For this review, take the finished solid that the model builds, in its own axes (mm). A direction names the side the tool comes from. Round coordinates to 2 decimals unless told otherwise and drop trailing zeros. Loops run counter-clockwise (first coordinate to the right, second up) from the corner with the lowest first, then second, coordinate; pieces in that order, holes last. Notation, with made-up numbers: (42, 23) -> (60, 23) arc R3 ccw to (60, 27) -> close; hole circle Ø3 at (27, 23.5). An arc over 180 degrees is marked (long way). Use one line per item in the form item = value. Start each with the question number.
from build123d import *

# Parameters (mm, degrees)
SKETCH1_W           = 40
SKETCH1_H           = 40
BOSS_EXTRUDE1_DEPTH = 40
SKETCH4_W           = 40
SKETCH4_H           = 40
CUT_EXTRUDE1_DEPTH  = 5
SKETCH5_W           = 40
SKETCH5_H           = 40
CUT_EXTRUDE2_DEPTH  = 5
SKETCH6_W           = 40
SKETCH6_H           = 40
CUT_EXTRUDE3_DEPTH  = 5
FILLET1_R           = 5
BOSS_EXTRUDE2_START = 5
BOSS_EXTRUDE2_DEPTH = 5
FILLET2_R           = 2.5
BOSS_EXTRUDE3_DEPTH = 0.1


with BuildPart() as part:
    # Sketch1 → Boss-Extrude1 (new body)
    with BuildSketch(Plane(origin=(0, 0, 0), x_dir=(0, 1, 0), z_dir=(0, 0, 1))):
        with Locations((20, -20)):
            Rectangle(SKETCH1_W, SKETCH1_H)
    extrude(amount=BOSS_EXTRUDE1_DEPTH)

    # Sketch2 → Cut-Revolve1 (revolve, cut)
    with BuildSketch(Plane.XZ):
        with BuildLine():
            Line((0, 42), (0, -42))
            ThreePointArc((0, -42), (42, 0), (0, 42))
        make_face()
    revolve(axis=Axis((0, 0, 42), (0, 0, -1)), mode=Mode.SUBTRACT)

    # Sketch4 → Cut-Extrude1 (cut)
    with BuildSketch(Plane.XZ):
        with Locations((20, 20)):
            Rectangle(SKETCH4_W, SKETCH4_H)
    extrude(amount=-CUT_EXTRUDE1_DEPTH, mode=Mode.SUBTRACT)

    # Sketch5 → Cut-Extrude2 (cut)
    with BuildSketch(Plane(origin=(0, 0, 0), x_dir=(0, -1, 0), z_dir=(-1, 0, 0))):
        with Locations((-20, 20)):
            Rectangle(SKETCH5_W, SKETCH5_H)
    extrude(amount=-CUT_EXTRUDE2_DEPTH, mode=Mode.SUBTRACT)

    # Sketch6 → Cut-Extrude3 (cut)
    with BuildSketch(Plane(origin=(0, 0, 0), x_dir=(1, 0, 0), z_dir=(0, 0, -1))):
        with Locations((20, -20)):
            Rectangle(SKETCH6_W, SKETCH6_H)
    extrude(amount=-CUT_EXTRUDE3_DEPTH, mode=Mode.SUBTRACT)

    # Fillet1
    fillet1_edges = [part.edges().sort_by_distance(p)[0] for p in [
        (22.5, 40, 40),
        (40, 22.5, 40),
        (40, 40, 22.5),
    ]]
    fillet(fillet1_edges, radius=FILLET1_R)

    # Sketch7 → Boss-Extrude2 (add)
    with BuildSketch(Plane.XZ.offset(-5).offset(BOSS_EXTRUDE2_START)):
        with BuildLine():
            Line((31.464466094, 40), (31.464466094, 35))
            Line((31.464466094, 35), (35, 31.464466094))
            Line((35, 31.464466094), (40, 31.464466094))
            Line((40, 31.464466094), (40, 35))
            ThreePointArc((40, 35), (38.535533906, 38.535533906), (35, 40))
            Line((35, 40), (31.464466094, 40))
        make_face()
    boss_extrude2 = extrude(amount=-BOSS_EXTRUDE2_DEPTH)

    # Mirror1: Boss-Extrude2 across plane
    add(boss_extrude2.mirror(Plane(origin=(0, 0, 0), x_dir=(0, 0.7071067811865476, 0.7071067811865476), z_dir=(0, 0.7071067811865477, -0.7071067811865475))))

    # Mirror1 at the second plane: Boss-Extrude2 across plane
    add(boss_extrude2.mirror(Plane(origin=(0, 0, 0), x_dir=(0, 0, 1), z_dir=(-0.7071067811865476, 0.7071067811865475, 0))))

    # Fillet2
    fillet2_edges = [part.edges().sort_by_distance(p)[0] for p in [
        (38.535533906, 0, 38.535533906),
        (33.232233047, 0, 40),
        (40, 0, 33.232233047),
        (0, 38.535533906, 38.535533906),
        (0, 40, 33.232233047),
        (0, 33.232233047, 40),
        (38.535533906, 38.535533906, 0),
        (40, 33.232233047, 0),
        (33.232233047, 40, 0),
    ]]
    fillet(fillet2_edges, radius=FILLET2_R)

    # Sketch9 → Boss-Extrude3 (add)
    with BuildSketch(Plane.YZ.offset(40)):
        with BuildLine():
            Line((32.5, 35), (5, 35))
            ThreePointArc((5, 35), (3.232233047, 34.267766953), (2.5, 32.5))
            Line((2.5, 32.5), (2.5, 10))
            ThreePointArc((2.5, 10), (4.696699141, 4.696699141), (10, 2.5))
            Line((10, 2.5), (32.5, 2.5))
            ThreePointArc((32.5, 2.5), (34.267766953, 3.232233047), (35, 5))
            Line((35, 5), (35, 32.5))
            ThreePointArc((35, 32.5), (34.267766953, 34.267766953), (32.5, 35))
        make_face()
    boss_extrude3 = extrude(amount=BOSS_EXTRUDE3_DEPTH)

    # Mirror2: Boss-Extrude3 across plane
    add(boss_extrude3.mirror(Plane(origin=(0, 0, 0), x_dir=(0.7071067811865475, 0, 0.7071067811865476), z_dir=(0.7071067811865478, 0, -0.7071067811865474))))

    # Mirror2 at the second plane: Boss-Extrude3 across plane
    add(boss_extrude3.mirror(Plane(origin=(0, 0, 0), x_dir=(0, 0, 1), z_dir=(-0.7071067811865476, 0.7071067811865475, 0))))


solid = part.part
Item 1: Wall thickness on line 1 (X direction, y = 29.5, z = 34); line 2 (Z direction, x = 34, y = 35); line 3 (X direction, y = 20.5, z = 7): over which ranges is each line inside the solid? List them lowest first.
Item 2: Machinability: for faces 1 (the flat face through (40, 34.4, 3)), 2 (the flat face through (31, 31, 5)), 3 (the flat face through (3.1, 34.5, 40)), 4 (the flat face through (40, 34.5, 34.5)), which of the approach directions +Z, -Z, +X, -X, +Y, -Y give a long, thin tool a straight path to every point of the face, cutting with its end or side? Answer none if there is none.
Item 3: Draft analysis for pull direction Y (two halves, no side actions). For faces 5 (the flat face through (31.464, 38, 2)), 6 (the flat face through (34, 0, 35)), 7 (the cylindrical face through (33.207, 39.287, 0.752)), state which applies: +Y half, -Y half, draft (parallel to the pull), parting line (faces both ways), or undercut.
Item 4: Take a section at B-B on y = 24. Give the boundary of the cut face in (x, z), plus the area to 3 significant figures.
Item 5: Take a section at A-A on z = 7. Give the boundary of the cut face in (x, y).
Item 6: Take a section at D-D on x = 9. Give the boundary of the cut face in (y, z), plus the area to 3 significant figures.
Item 7: Take a section at C-C on x = 15. Give the boundary of the cut face in (y, z), plus the area to 3 significant figures.
Item 8: For P1, Ø10, axis at x = 22, y = 12, coming from the -Z side; P2, Ø1.5, axis at y = 21, z = 10, coming from the -X side, all flat-tipped, find the tip position at first contact; note any pin that passes through.
Results:
q1.line_1 = 5 to 40.1
q1.line_2 = 0 to 40
q1.line_3 = 35.98 to 40.1
q2.face_1 = -Z, +X, +Y
q2.face_2 = -Z, -X, -Y
q2.face_3 = +Z, -X, +Y
q2.face_4 = +Z, +X, +Y
q3.face_5 = draft
q3.face_6 = -Y half
q3.face_7 = +Y half
q4.outline = (2.5, 40) -> (5, 40) -> (5, 34.1) arc R34.47 cw to (34.1, 5) -> (40, 5) -> (40, 2.5) -> (40.1, 2.5) -> (40.1, 35) -> (40, 35) arc R5 ccw to (35, 40) -> (35, 40.1) -> (2.5, 40.1) -> close
q4.area = 612 mm2
q5.outline = (3.13, 40) -> (10.72, 40) arc R41.41 cw to (40, 10.72) -> (40, 3.13) -> (40.1, 3.13) -> (40.1, 35) -> (40, 35) arc R5 ccw to (35, 40) -> (35, 40.1) -> (3.13, 40.1) -> close
q6.outline = (2.57, 40) -> (9.11, 40) arc R41.02 cw to (40, 9.11) -> (40, 2.57) -> (40.1, 2.57) -> (40.1, 35) -> (40, 35) arc R5 ccw to (35, 40) -> (35, 40.1) -> (2.57, 40.1) -> close
q6.area = 292 mm2
q7.outline = (2.5, 40) -> (5, 40) -> (5, 38.91) arc R39.23 cw to (38.91, 5) -> (40, 5) -> (40, 2.5) -> (40.1, 2.5) -> (40.1, 35) -> (40, 35) arc R5 ccw to (35, 40) -> (35, 40.1) -> (2.5, 40.1) -> close
q7.area = 384 mm2
q8.P1 = 29.33
q8.P2 = 34.46
